Part model, mm, in its own coordinate system. Coordinates: 2 decimals unless noted, no trailing zeros. Loops run counter-clockwise (first coordinate to the right, second up) from the corner with the lowest first, then second, coordinate; pieces in that order, holes last. Notation, with made-up numbers: M 70,74.25 L 106,74.25 A22 ccw 106,109.25 Z; hole C 32.5,-7.75 d1. An arc over 180 degrees is marked long. Use a Markdown table: item, result. Add a question column.
1) Band-saw the part on B-B (y = 3). List the corners of the cut face in (x, z), plus the area to 3 significant figures.
2) Pin check, flat tip, straight feed: pin 1 Ø1.4 at (x, y) = (-3.6, -3) entering from +Z. Stop position of the tip, or through.
3) Wall check: probe 1 along Y at (x, z) = (3.25, 0.2) (3 decimals); probe 2 along Y at (x, z) = (3.5, 0.6); probe 3 along X at (y, z) = (3.5, 0.4). Give the ranges that are in metal, low to high. Write a range as from..to.
4) Band-saw the part on C-C (z = 0.65). List the corners of the cut face in (x, y) (3 decimals), plus the area to 3 significant figures.
5) Band-saw the part on A-A (x = -3). List the corners of the cut face in (y, z).
6) Pull direction X, two halves, no side cores. Call faces 1 (the flat face through (1, -1, 0.8)), 2 (the cylindrical face through (2.85, 3.03, 0.41)), 3 (the cylindrical face through (-1.801, 0.285, 0.394)), 4 (the cylindrical face through (-4.35, -2.97, 0.41)): released by +X, released by -X, zero draft, split by the parting line, or undercut.
7) Band-saw the part on D-D (x = 3.25). List the corners of the cut face in (y, z) (3 decimals), plus the area to 3 significant figures.
from build123d import *

# Parameters (mm, degrees)
SKETCH_1_W          = 12
SKETCH_1_H          = 10
EXTRUDE_1_DEPTH     = 0.8
CUT_EXTRUDE_1_REACH = 9.851
SKETCH_2_R          = 0.375
SKETCH_2_R_2        = 0.75
SKETCH_2_W          = 4.5
SKETCH_2_H          = 5
FILLET_1_R          = 1


with BuildPart() as part:
    # Эскиз1 → Бобышка-Вытянуть1 (new body)
    with BuildSketch(Plane.XY):
        Rectangle(SKETCH_1_W, SKETCH_1_H)
    extrude(amount=EXTRUDE_1_DEPTH)

    # Эскиз2 → Вырез-Вытянуть1 (cut, up to next)
    with BuildSketch(Plane.XY.offset(0.8), mode=Mode.PRIVATE) as cut_extrude_1_sk1:
        Circle(SKETCH_2_R)
    cut_extrude_1_tool1 = extrude(cut_extrude_1_sk1.sketch, amount=-CUT_EXTRUDE_1_REACH, mode=Mode.PRIVATE) & part.part
    # Эскиз2 → Вырез-Вытянуть1 (cut, up to next)
    with BuildSketch(Plane.XY.offset(0.8), mode=Mode.PRIVATE) as cut_extrude_1_sk2:
        with Locations((-3.6, -3)):
            Circle(SKETCH_2_R_2)
    cut_extrude_1_tool2 = extrude(cut_extrude_1_sk2.sketch, amount=-CUT_EXTRUDE_1_REACH, mode=Mode.PRIVATE) & part.part
    # Эскиз2 → Вырез-Вытянуть1 (cut, up to next)
    with BuildSketch(Plane.XY.offset(0.8), mode=Mode.PRIVATE) as cut_extrude_1_sk3:
        with Locations((3.6, 3)):
            Circle(SKETCH_2_R_2)
    cut_extrude_1_tool3 = extrude(cut_extrude_1_sk3.sketch, amount=-CUT_EXTRUDE_1_REACH, mode=Mode.PRIVATE) & part.part
    # Эскиз2 → Вырез-Вытянуть1 (cut, up to next)
    with BuildSketch(Plane.XY.offset(0.8), mode=Mode.PRIVATE) as cut_extrude_1_sk4:
        with Locations((3.25, -2)):
            Circle(SKETCH_2_R)
    cut_extrude_1_tool4 = extrude(cut_extrude_1_sk4.sketch, amount=-CUT_EXTRUDE_1_REACH, mode=Mode.PRIVATE) & part.part
    # Эскиз2 → Вырез-Вытянуть1 (cut, up to next)
    with BuildSketch(Plane.XY.offset(0.8), mode=Mode.PRIVATE) as cut_extrude_1_sk5:
        with Locations((-3.75, 2.5)):
            Rectangle(SKETCH_2_W, SKETCH_2_H)
    cut_extrude_1_tool5 = extrude(cut_extrude_1_sk5.sketch, amount=-CUT_EXTRUDE_1_REACH, mode=Mode.PRIVATE) & part.part
    add(cut_extrude_1_tool1.solids().sort_by_distance((0, 0, 0.8))[0], mode=Mode.SUBTRACT)
    add(cut_extrude_1_tool2.solids().sort_by_distance((-3.6, -3, 0.8))[0], mode=Mode.SUBTRACT)
    add(cut_extrude_1_tool3.solids().sort_by_distance((3.6, 3, 0.8))[0], mode=Mode.SUBTRACT)
    add(cut_extrude_1_tool4.solids().sort_by_distance((3.25, -2, 0.8))[0], mode=Mode.SUBTRACT)
    add(cut_extrude_1_tool5.solids().sort_by_distance((-3.75, 2.5, 0.8))[0], mode=Mode.SUBTRACT)

    # Скругление1
    fillet_1_edges = [part.edges().sort_by_distance(p)[0] for p in [
        (-6, 0, 0.4),
        (-1.5, 5, 0.4),
        (-1.5, 0, 0.4),
        (6, -5, 0.4),
        (-6, -5, 0.4),
        (6, 5, 0.4),
    ]]
    fillet(fillet_1_edges, radius=FILLET_1_R)


solid = part.part
Entries:
| question | item | result |
|---|---|---|
| 1 | outline | M -1.5,0 L 2.85,0 L 2.85,0.8 L -1.5,0.8 Z; M 4.35,0 L 6,0 L 6,0.8 L 4.35,0.8 Z |
| 1 | area | 4.80 mm2 |
| 2 | pin 1 | through |
| 3 | probe 1 | -5..-2.375, -1.625..2.337, 3.663..5 |
| 3 | probe 2 | -5..-2.28, -1.72..2.26, 3.74..5 |
| 3 | probe 3 | -1.5..3.04, 4.16..6 |
| 4 | outline | M -6,-4 A1 ccw -5,-5 L 5,-5 A1 ccw 6,-4 L 6,4 A1 ccw 5,5 L -0.5,5 A1 ccw -1.5,4 L -1.5,1 A1 cw -2.5,0 L -5,0 A1 ccw -6,-1 Z; hole C -3.6,-3 d1.5; hole C 0,0 d0.75; hole C 3.6,3 d1.5; hole C 3.25,-2 d0.75 |
| 4 | area | 92.2 mm2 |
| 5 | outline | M -5,0 L -3.45,0 L -3.45,0.8 L -5,0.8 Z; M -2.55,0 L 0,0 L 0,0.8 L -2.55,0.8 Z |
| 6 | face 1 | zero draft |
| 6 | face 2 | undercut |
| 6 | face 3 | released by -X |
| 6 | face 4 | undercut |
| 7 | outline | M -5,0 L -2.375,0 L -2.375,0.8 L -5,0.8 Z; M -1.625,0 L 2.337,0 L 2.337,0.8 L -1.625,0.8 Z; M 3.663,0 L 5,0 L 5,0.8 L 3.663,0.8 Z |
| 7 | area | 6.34 mm2 |
